Can you work these out from the model? Positions are in its coordinate system, mm. Face numbers are marked on the shaded views. A direction names the side the tool comes from. Round coordinates to 2 decimals unless told otherwise and drop trailing zeros. Order: outer loops, then holes, each group sorted by start corner. A loop starts at its lowest first (then second) coordinate and runs counter-clockwise, first axis right, second up. Notation, with made-up numbers: (-12.5, 19.5) - (16.5, 19.5) arc R8 ccw to (16.5, 29.5) - close; hole circle Ø6 at (61.25, -26). An arc over 180 degrees is marked (long way). Write item = value, one per line.
from build123d import *

# Parameters (mm, degrees)
SKETCH_1_R      = 10
SKETCH_1_R_2    = 5.1
EXTRUDE_1_DEPTH = 15
SKETCH_2_R      = 15
SKETCH_2_R_2    = 5
EXTRUDE_2_DEPTH = 2
SKETCH_3_R      = 9
SKETCH_3_R_2    = 5
EXTRUDE_3_DEPTH = 10
FILLET_1_R      = 2


with BuildPart() as part:
    # 草图1 → 凸台-拉伸1 (new body)
    with BuildSketch(Plane.XY):
        Circle(SKETCH_1_R)
        Circle(SKETCH_1_R_2, mode=Mode.SUBTRACT)
    extrude(amount=EXTRUDE_1_DEPTH)

    # 草图2 → 凸台-拉伸2 (add)
    with BuildSketch(Plane.XY.offset(15)):
        Circle(SKETCH_2_R)
        Circle(SKETCH_2_R_2, mode=Mode.SUBTRACT)
    extrude(amount=EXTRUDE_2_DEPTH)

    # 草图3 → 凸台-拉伸3 (add)
    with BuildSketch(Plane.XY.offset(17)):
        Circle(SKETCH_3_R)
        Circle(SKETCH_3_R_2, mode=Mode.SUBTRACT)
    extrude(amount=EXTRUDE_3_DEPTH)

    # 圆角1
    fillet_1_edges = [part.edges().sort_by_distance(p)[0] for p in [
        (-9, 0, 17),
        (-9, 0, 27),
        (-5, 0, 27),
        (-10, 0, 0),
    ]]
    fillet(fillet_1_edges, radius=FILLET_1_R - 0.0001)  # a hair under: the kernel refuses the full size


solid = part.part
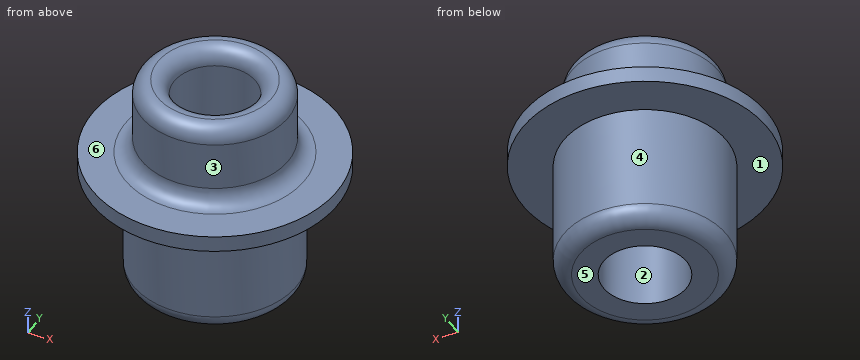
(1) If we section it at C-C (z = 5.25): Write out the boundary of the cut face in (x, y), plus the area to 3 significant figures.
Computed:
outline = circle Ø20 at (0, 0); hole circle Ø10.2 at (0, 0)
area = 232 mm^2
(2) If we section it at D-D (y = -12.25): Write out the boundary of the cut face in (x, z).
Computed:
outline = (-8.66, 15) - (8.66, 15) - (8.66, 17) - (-8.66, 17) - close
(3) Thinking about a two-plate mould opening in X: for the marked faces 1, 2 and 3, which applies, +X half, -X half, draft (parallel to the pull), parting line (faces both ways), or undercut?
Computed:
face_1 = draft
face_2 = undercut
face_3 = parting line
(4) Will these pins go through, and if not, where does the flat tip stop? P1, Ø11.5, axis at x = 0, y = 0, coming from the +Z side; P2, Ø4, axis at y = 10.5, z = 3, coming from the -X side; P3, Ø3, axis at x = -5, y = -0.5, coming from the +Z side.
Computed:
P1 = 26.56
P2 = -5.27
P3 = 26.94
(5) If I drill on line 1 (Y direction, x = 0, z = 21.25); line 2 (Y direction, x = 0, z = 4.75); line 3 (Z direction, x = -11, y = -7.75), over which ranges is the centre line in solid material (lowest first)? Write a range as from..to.
Computed:
line_1 = -9..-5, 5..9
line_2 = -10..-5.1, 5.1..10
line_3 = 15..17
(6) On a 3-axis mill with a long thin cutter (end or side, diameter ignored), from which of +Z, -Z, +X, -X, +Y, -Y can I reach the whole of each face in a straight line? I mean the marked faces 4, 5 and 6. Say none if no direction works.
Computed:
face_4 = -Z
face_5 = -Z, +X, -X, +Y, -Y
face_6 = +Z
